from build123d import *


with BuildPart() as part:
    # Sketch1 → Revolve1 (revolve)
    with BuildSketch(Plane(origin=(0, 0, 0), x_dir=(0, 0, -1), z_dir=(1, 0, 0))):
        with BuildLine():
            Line((0, -12.118048154), (0, -15.348048154))
            Line((0, -15.348048154), (-16.15, -15.348048154))
            ThreePointArc((-16.15, -15.348048154), (-17.564213562, -14.762261716), (-18.15, -13.348048154))
            Line((-18.15, -13.348048154), (-18.15, -7.718048154))
            ThreePointArc((-18.15, -7.718048154), (-17.564213562, -6.303834591), (-16.15, -5.718048154))
            Line((-16.15, -5.718048154), (-6, -5.718048154))
            Line((-6, -5.718048154), (-6, -9.618048154))
            Line((-6, -9.618048154), (-14.25, -9.618048154))
            Line((-14.25, -9.618048154), (-14.25, -12.118048154))
            Line((-14.25, -12.118048154), (0, -12.118048154))
        make_face()
    revolve(axis=Axis((0, 41.234250563, 0), (0, -1, 0)))


solid = part.part
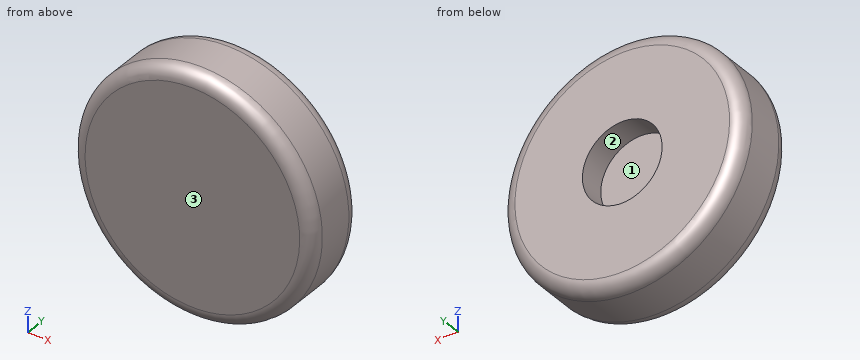
Input: part model. Units: mm. Frame: model coordinates. Face numbers are marked on the shaded views. Coordinates: 2 decimals unless noted, no trailing zeros. Order: outer loops, then holes, each group sorted by start corner. A loop starts at its lowest first (then second) coordinate and runs counter-clockwise, first axis right, second up. Notation, with made-up numbers: M 63,84 L 80,84 A17 ccw 80,107 Z; hole C 5,6.25 d2. An arc over 180 degrees is marked long. Answer as CSV lines item,"result".
1. Section B-B (z = 0). Return the cut outline in (x, y), then the cut area to 3 significant figures.
Reported:
outline,"M -18.15,-13.35 A2 ccw -16.15,-15.35 L 16.15,-15.35 A2 ccw 18.15,-13.35 L 18.15,-7.72 A2 ccw 16.15,-5.72 L 6,-5.72 L 6,-9.62 L 14.25,-9.62 L 14.25,-12.12 L -14.25,-12.12 L -14.25,-9.62 L -6,-9.62 L -6,-5.72 L -16.15,-5.72 A2 ccw -18.15,-7.72 Z"
area,"228 mm2"
2. Section A-A (x = 0). Return the cut outline in (y, z), then the cut area to 3 significant figures.
Reported:
outline,"M -15.35,-16.15 A2 ccw -13.35,-18.15 L -7.72,-18.15 A2 ccw -5.72,-16.15 L -5.72,-6 L -9.62,-6 L -9.62,-14.25 L -12.12,-14.25 L -12.12,14.25 L -9.62,14.25 L -9.62,6 L -5.72,6 L -5.72,16.15 A2 ccw -7.72,18.15 L -13.35,18.15 A2 ccw -15.35,16.15 Z"
area,"228 mm2"
3. Material intervals for line 1 (X direction, y = -8.65, z = 0); line 2 (Y direction, x = -11.5, z = 3.5); line 3 (X direction, y = -11.45, z = 0), sorted ascending. Write a range as from..to.
Reported:
line 1,"-18.15..-6, 6..18.15"
line 2,"-15.35..-12.12, -9.62..-5.72"
line 3,"-18.15..-14.25, 14.25..18.15"
4. Pull-direction query (Y, two-part tool) for the marked faces 1, 2 and 3; classes: released by +Y, released by -Y, zero draft, split by the parting line, or undercut.
Reported:
face 1,"undercut"
face 2,"zero draft"
face 3,"released by -Y"
5. Section C-C (y = -10.5). Return the cut outline in (x, z), then the cut area to 3 significant figures.
Reported:
outline,"C 0,0 d36.3; hole C 0,0 d28.5"
area,"397 mm2"
